Design review of the part built by this model. Coordinates are the model's own, in mm. A direction names the side the tool comes from. Coordinates: 2 decimals unless noted, no trailing zeros. Write each loop counter-clockwise with the first axis right and the second up, starting at its lowest first coordinate (ties: lowest second). Pieces come first, ordered by that corner, then holes. Notation, with made-up numbers: M 11.25,89 L 33.25,89 A14 cw 33.25,111 Z; hole C -13.5,-26.75 d9. An arc over 180 degrees is marked long. One line per question, with ' | ' between items.
from build123d import *

# Parameters (mm, degrees)
SKETCH_2_W                       = 89.1
SKETCH_2_H                       = 1.5
SM_BASE_FLANGE_1_DEPTH           = 152
SM_EDGE_FLANGE_1_STRIP_W         = 7.4732
SM_EDGE_FLANGE_1_STRIP_H         = 1.5
SM_EDGE_FLANGE_1_STRIP_CUT_DEPTH = 152
SM_EDGE_FLANGE_1_DEPTH           = 152
SM_EDGE_FLANGE_2_STRIP_W         = 7.4732
SM_EDGE_FLANGE_2_STRIP_H         = 1.5
SM_EDGE_FLANGE_2_STRIP_CUT_DEPTH = 152
SM_EDGE_FLANGE_2_DEPTH           = 152
SKETCH_13_W                      = 16.114616681
SKETCH_13_H                      = 12.6
SKETCH_13_W_2                    = 14.895249376
CUT_EXTRUDE_1_DEPTH              = 177.473255764
SM_EDGE_FLANGE_3_STRIP_W         = 7.4732
SM_EDGE_FLANGE_3_STRIP_H         = 1.5
SM_EDGE_FLANGE_3_STRIP_CUT_DEPTH = 84.6268
SM_EDGE_FLANGE_3_DEPTH           = 84.6268
SKETCH_17_R                      = 2.25
CUT_EXTRUDE_2_DEPTH              = 10
SKETCH_18_R                      = 2.25
CUT_EXTRUDE_3_DEPTH              = 10
SKETCH_19_W                      = 28
SKETCH_19_H                      = 40
CUT_EXTRUDE_4_DEPTH              = 10
SM_START                         = 89.75
SM_EDGE_FLANGE_4_DEPTH           = 41.5
SM_EDGE_FLANGE_4_2_DEPTH         = 0.75
SM_START_2                       = 130.5
SM_EDGE_FLANGE_4_3_DEPTH         = 0.75
SM_START_3                       = 90.5
SM_EDGE_FLANGE_4_4_DEPTH         = 40
HOLE_WIZARD_M3_1_D               = 2.5
HOLE_WIZARD_M3_1_DEPTH           = 7.5
HOLE_WIZARD_M3_1_TIP             = 0.751075774
HOLE_WIZARD_M4_1_D               = 3.3
HOLE_WIZARD_M4_1_DEPTH           = 10.1
HOLE_WIZARD_M4_1_TIP             = 0.991420021
SKETCH_27_R                      = 1.5
CUT_EXTRUDE_5_DEPTH              = 20
SKETCH_28_R                      = 1.5
CUT_EXTRUDE_6_DEPTH              = 10
CUT_EXTRUDE_START                = -0.75
SKETCH_29_W                      = 28
SKETCH_29_H                      = 1.5
CUT_EXTRUDE_7_DEPTH              = 0.75
SKETCH_30_W                      = 28
SKETCH_30_H                      = 1.5
CUT_EXTRUDE_8_DEPTH              = 0.75


# Read off the part's stored shape, not the designer's step: 边线-法兰4
# Sheet-metal steps are written as plain solids
with BuildPart() as part:
    # Sketch 2 → 基体-法兰1 (new body)
    with BuildSketch(Plane.XY):
        with Locations((44.55, -0.75)):
            Rectangle(SKETCH_2_W, SKETCH_2_H)
    extrude(amount=SM_BASE_FLANGE_1_DEPTH)

    # 边线-法兰1 strip (across the edge) → 边线-法兰1 strip cut (cut)
    with BuildSketch(Plane.XY):
        with Locations((-1.5, -0.75)):
            Rectangle(SM_EDGE_FLANGE_1_STRIP_W, SM_EDGE_FLANGE_1_STRIP_H)
    extrude(amount=SM_EDGE_FLANGE_1_STRIP_CUT_DEPTH, mode=Mode.SUBTRACT)

    # 边线-法兰1 section (across the edge) → 边线-法兰1 (add)
    with BuildSketch(Plane.XY):
        with BuildLine():
            Line((0, 0.7366), (0, 8.5))
            Line((0, 8.5), (1.5, 8.5))
            Line((1.5, 8.5), (1.5, 0.7366))
            ThreePointArc((1.5, 0.7366), (1.715745145, 0.215745145), (2.2366, 0))
            Line((2.2366, 0), (2.2366, -1.5))
            ThreePointArc((2.2366, -1.5), (0.655084973, -0.844915027), (0, 0.7366))
        make_face()
    extrude(amount=SM_EDGE_FLANGE_1_DEPTH)

    # 边线-法兰2 strip (across the edge) → 边线-法兰2 strip cut (cut)
    with BuildSketch(Plane(origin=(89.1, 0, 152), x_dir=(-1, 0, 0), z_dir=(0, 0, -1))):
        with Locations((-1.5, -0.75)):
            Rectangle(SM_EDGE_FLANGE_2_STRIP_W, SM_EDGE_FLANGE_2_STRIP_H)
    extrude(amount=SM_EDGE_FLANGE_2_STRIP_CUT_DEPTH, mode=Mode.SUBTRACT)

    # 边线-法兰2 section (across the edge) → 边线-法兰2 (add)
    with BuildSketch(Plane(origin=(89.1, 0, 152), x_dir=(-1, 0, 0), z_dir=(0, 0, -1))):
        with BuildLine():
            Line((0, 0.7366), (0, 8.5))
            Line((0, 8.5), (1.5, 8.5))
            Line((1.5, 8.5), (1.5, 0.7366))
            ThreePointArc((1.5, 0.7366), (1.715745145, 0.215745145), (2.2366, 0))
            Line((2.2366, 0), (2.2366, -1.5))
            ThreePointArc((2.2366, -1.5), (0.655084973, -0.844915027), (0, 0.7366))
        make_face()
    extrude(amount=SM_EDGE_FLANGE_2_DEPTH)

    # 草图13 → 切除-拉伸1 (cut, through all)
    with BuildSketch(Plane.XZ.offset(1.5)):
        with Locations((-5.82070834, 145.7)):
            Rectangle(SKETCH_13_W, SKETCH_13_H)
        with Locations((94.311024688, 145.7)):
            Rectangle(SKETCH_13_W_2, SKETCH_13_H)
    extrude(amount=-CUT_EXTRUDE_1_DEPTH, mode=Mode.SUBTRACT)

    # 边线-法兰3 strip (across the edge) → 边线-法兰3 strip cut (cut)
    with BuildSketch(Plane(origin=(86.8634, -1.5, 152), x_dir=(0, 0, -1), z_dir=(-1, 0, 0))):
        with Locations((-1.5, -0.75)):
            Rectangle(SM_EDGE_FLANGE_3_STRIP_W, SM_EDGE_FLANGE_3_STRIP_H)
    extrude(amount=SM_EDGE_FLANGE_3_STRIP_CUT_DEPTH, mode=Mode.SUBTRACT)

    # 边线-法兰3 section (across the edge) → 边线-法兰3 (add)
    with BuildSketch(Plane(origin=(86.8634, -1.5, 152), x_dir=(0, 0, -1), z_dir=(-1, 0, 0))):
        with BuildLine():
            Line((0, 0.7366), (0, 8.5))
            Line((0, 8.5), (1.5, 8.5))
            Line((1.5, 8.5), (1.5, 0.7366))
            ThreePointArc((1.5, 0.7366), (1.715745145, 0.215745145), (2.2366, 0))
            Line((2.2366, 0), (2.2366, -1.5))
            ThreePointArc((2.2366, -1.5), (0.655084973, -0.844915027), (0, 0.7366))
        make_face()
    extrude(amount=SM_EDGE_FLANGE_3_DEPTH)

    # 草图17 → 切除-拉伸2 (cut)
    with BuildSketch(Plane.XY.offset(152)):
        with Locations((80.55, -6)):
            Circle(SKETCH_17_R)
        with Locations(Location((8.55, -6, 0), (0, 0, 270))):
            Circle(SKETCH_17_R)
    extrude(amount=-CUT_EXTRUDE_2_DEPTH, mode=Mode.SUBTRACT)

    # 草图18 → 切除-拉伸3 (cut)
    with BuildSketch(Plane.XZ.offset(1.5)):
        with Locations(Location((17.05, 145.5, 0), (0, 0, 270))):
            Circle(SKETCH_18_R)
        with Locations(Location((72.05, 145.5, 0), (0, 0, 90))):
            Circle(SKETCH_18_R)
    extrude(amount=-CUT_EXTRUDE_3_DEPTH, mode=Mode.SUBTRACT)

    # 草图19 → 切除-拉伸4 (cut)
    with BuildSketch(Plane.XZ.offset(1.5)):
        with Locations((34.3, 110.5)):
            Rectangle(SKETCH_19_W, SKETCH_19_H)
    extrude(amount=-CUT_EXTRUDE_4_DEPTH, mode=Mode.SUBTRACT)

    # 边线-法兰4 outline → 边线-法兰4 (cut)
    with BuildSketch(Plane.XY.offset(SM_START)):
        with BuildLine():
            Line((20.3, -1.5), (20.3, 0))
            Line((20.3, 0), (18.0634, 0))
            ThreePointArc((18.0634, 0), (19.358564082, -0.413161062), (20.175223856, -1.5))
            Line((20.175223856, -1.5), (20.3, -1.5))
        make_face()
    extrude(amount=SM_EDGE_FLANGE_4_DEPTH, mode=Mode.SUBTRACT)

    # Sm Edge Flange 4 2 outline → Sm Edge Flange 4 2 (cut)
    with BuildSketch(Plane.XY.offset(SM_START)):
        with BuildLine():
            ThreePointArc((20.175223856, -1.5), (19.358564082, -0.413161062), (18.0634, 0))
            Line((18.0634, 0), (17.3134, 0))
            Line((17.3134, 0), (17.3134, -1.5))
            Line((17.3134, -1.5), (20.175223856, -1.5))
        make_face()
    extrude(amount=SM_EDGE_FLANGE_4_2_DEPTH, mode=Mode.SUBTRACT)

    # Sm Edge Flange 4 3 outline → Sm Edge Flange 4 3 (cut)
    with BuildSketch(Plane.XY.offset(SM_START_2)):
        with BuildLine():
            ThreePointArc((20.175223856, -1.5), (19.358564082, -0.413161062), (18.0634, 0))
            Line((18.0634, 0), (17.3134, 0))
            Line((17.3134, 0), (17.3134, -1.5))
            Line((17.3134, -1.5), (20.175223856, -1.5))
        make_face()
    extrude(amount=SM_EDGE_FLANGE_4_3_DEPTH, mode=Mode.SUBTRACT)

    # Sm Edge Flange 4 4 outline → Sm Edge Flange 4 4 (add)
    with BuildSketch(Plane.XY.offset(SM_START_3)):
        with BuildLine():
            ThreePointArc((20.3, -2.2366), (20.268585343, -1.863053267), (20.175223856, -1.5))
            Line((20.175223856, -1.5), (18.0634, -1.5))
            ThreePointArc((18.0634, -1.5), (18.584254855, -1.715745145), (18.8, -2.2366))
            Line((18.8, -2.2366), (18.8, -25))
            Line((18.8, -25), (20.3, -25))
            Line((20.3, -25), (20.3, -2.2366))
        make_face()
    extrude(amount=SM_EDGE_FLANGE_4_4_DEPTH)

    # M3 螺纹孔1
    with Locations(Plane.ZY.offset(-18.8)):
        with Locations((101.5, -20), (120.5, -20)):
            Hole(HOLE_WIZARD_M3_1_D / 2, depth=HOLE_WIZARD_M3_1_DEPTH)
            with Locations((0, 0, -(HOLE_WIZARD_M3_1_DEPTH + HOLE_WIZARD_M3_1_TIP / 2))):  # 118° drill point
                Cone(0, HOLE_WIZARD_M3_1_D / 2, HOLE_WIZARD_M3_1_TIP, mode=Mode.SUBTRACT)

    # M4 螺纹孔1
    with Locations(Plane.ZY):
        with Locations((30, 4.5)):
            Hole(HOLE_WIZARD_M4_1_D / 2, depth=HOLE_WIZARD_M4_1_DEPTH)
            with Locations((0, 0, -(HOLE_WIZARD_M4_1_DEPTH + HOLE_WIZARD_M4_1_TIP / 2))):  # 118° drill point
                Cone(0, HOLE_WIZARD_M4_1_D / 2, HOLE_WIZARD_M4_1_TIP, mode=Mode.SUBTRACT)

    # 草图27 → 切除-拉伸5 (cut)
    with BuildSketch(Plane(origin=(20.3, 0, 0), x_dir=(0, 0, -1), z_dir=(1, 0, 0))):
        with Locations(Location((-121.5, -9, 0), (0, 0, 90))):
            Circle(SKETCH_27_R)
    extrude(amount=-CUT_EXTRUDE_5_DEPTH, mode=Mode.SUBTRACT)

    # 草图28 → 切除-拉伸6 (cut)
    with BuildSketch(Plane(origin=(20.3, 0, 0), x_dir=(0, 0, -1), z_dir=(1, 0, 0))):
        with Locations(Location((-124.5, -5, 0), (0, 0, 90))):
            Circle(SKETCH_28_R)
    extrude(amount=-CUT_EXTRUDE_6_DEPTH, mode=Mode.SUBTRACT)

    # 草图29 → 切除-拉伸7 (cut)
    with BuildSketch(Plane.XY.offset(90.5).offset(CUT_EXTRUDE_START)):
        with Locations((34.3, -0.75)):
            Rectangle(SKETCH_29_W, SKETCH_29_H)
    extrude(amount=CUT_EXTRUDE_7_DEPTH, mode=Mode.SUBTRACT)

    # 草图30 → 切除-拉伸8 (cut)
    with BuildSketch(Plane(origin=(0, 0, 130.5), x_dir=(-1, 0, 0), z_dir=(0, 0, -1)).offset(CUT_EXTRUDE_START)):
        with Locations((-34.3, -0.75)):
            Rectangle(SKETCH_30_W, SKETCH_30_H)
    extrude(amount=CUT_EXTRUDE_8_DEPTH, mode=Mode.SUBTRACT)


solid = part.part
1. To check wall thickness, follow line 1 along Z through (x, y) = (19.1, -9); line 2 along X through (y, z) = (-0.3, 145.5); line 3 along Z through (x, y) = (19, -5). State the ranges of each line that lie inside material, in increasing order. Write a range as [from, to].
Answer sheet:
line 1: [90.5, 120], [123, 130.5], [150.5, 152] | line 2: [2.24, 14.8], [19.3, 69.8], [74.3, 86.86] | line 3: [90.5, 123], [126, 130.5], [150.5, 152]
2. Take a section at A-A (x = 42.5). Write out the cut boundary in (y, z).
Answer sheet:
outline: M -10,150.5 L -2.24,150.5 A0.74 cw -1.5,149.76 L -1.5,131.25 L 0,131.25 L 0,149.76 A2.24 ccw -2.24,152 L -10,152 Z; M -1.5,0 L 0,0 L 0,89.75 L -1.5,89.75 Z
3. Take a section at C-C (z = 56.5). Write out the cut boundary in (x, y), then the cut area to 3 significant figures.
Answer sheet:
outline: M 0,0.74 A2.24 ccw 2.24,-1.5 L 86.86,-1.5 A2.24 ccw 89.1,0.74 L 89.1,8.5 L 87.6,8.5 L 87.6,0.74 A0.74 cw 86.86,0 L 2.24,0 A0.74 cw 1.5,0.74 L 1.5,8.5 L 0,8.5 Z | area: 157 mm^2
4. Insertion check: pin 1 Ø5 at (x, z) = (72.05, 145.5) entering from +Y; pin 2 Ø2 at (y, z) = (-20, 101.5) entering from +X; pin 3 Ø10 at (x, z) = (40.5, 37) entering from -Y; pin 4 Ø0.9 at (x, y) = (19.5, -11) entering from -Z. Each pin has a flat end and moves straight along its axis. Give the tip position at first contact, or say it passes through.
Answer sheet:
pin 1: y = 0 | pin 2: through | pin 3: y = -1.5 | pin 4: z = 90.5
5. Draft analysis for pull direction Y (two halves, no side actions). For faces 1 (the face through (0.76, 3.5, 31.31)), 2 (the face through (2.237, -1, 148)), 3 (the face through (44, 0, 74)), state which applies: pulls with the +Y half, pulls with the -Y half, needs draft (parallel to the pull), parting line crosses it, or undercut.
Answer sheet:
face 1: undercut | face 2: needs draft | face 3: pulls with the +Y half
6. Take a section at D-D (x = 80.55). Write out the cut boundary in (y, z).
Answer sheet:
outline: M -10,150.5 L -8.25,150.5 L -8.25,152 L -10,152 Z; M -3.75,150.5 L -2.24,150.5 A0.74 cw -1.5,149.76 L -1.5,0 L 0,0 L 0,149.76 A2.24 ccw -2.24,152 L -3.75,152 Z
7. Take a section at B-B (x = 61.5). Write out the cut boundary in (y, z).
Answer sheet:
outline: M -10,150.5 L -2.24,150.5 A0.74 cw -1.5,149.76 L -1.5,0 L 0,0 L 0,149.76 A2.24 ccw -2.24,152 L -10,152 Z
8. Tool access review of faces 4 (the face through (87.6, 5, 71)), 5 (the face through (20.3, -14, 110)), 6 (the face through (86.863, -1, 148)), 7 (the face through (18.8, -13, 110)), 8 (the face through (19, -12, 90.5)): name each direction out of +Z, -Z, +X, -X, +Y, -Y from which nothing blocks a thin tool from reaching the whole face with its end or side.
Answer sheet:
face 4: +Z, -Z, +Y | face 5: -Z, +X, +Y, -Y | face 6: +Z, +X, +Y, -Y | face 7: -Z, -X, -Y | face 8: +Y, -Y
